from build123d import *

# Parameters (mm, degrees)
SKETCH_1_R      = 7.5
SKETCH_1_R_2    = 5
EXTRUDE_1_DEPTH = 4
SKETCH_2_R      = 8.25
SKETCH_2_R_2    = 7.5
EXTRUDE_2_DEPTH = 0.8
CHAMFER_1_SIZE  = 0.2


with BuildPart() as part:
    # 草图1 → 凸台-拉伸1 (new body)
    with BuildSketch(Plane.XY):
        Circle(SKETCH_1_R)
        Circle(SKETCH_1_R_2, mode=Mode.SUBTRACT)
    extrude(amount=EXTRUDE_1_DEPTH)

    # 草图2 → 凸台-拉伸2 (add)
    with BuildSketch(Plane(origin=(0, 0, 0), x_dir=(-1, 0, 0), z_dir=(0, 0, -1))):
        Circle(SKETCH_2_R)
        Circle(SKETCH_2_R_2, mode=Mode.SUBTRACT)
    extrude(amount=-EXTRUDE_2_DEPTH)

    # 倒角1
    chamfer_1_edges = [part.edges().sort_by_distance(p)[0] for p in [
        (8.25, 0, 0.8),
        (8.25, 0, 0),
        (-7.5, 0, 4),
        (-5, 0, 0),
        (-5, 0, 4),
    ]]
    chamfer(chamfer_1_edges, length=CHAMFER_1_SIZE)


solid = part.part
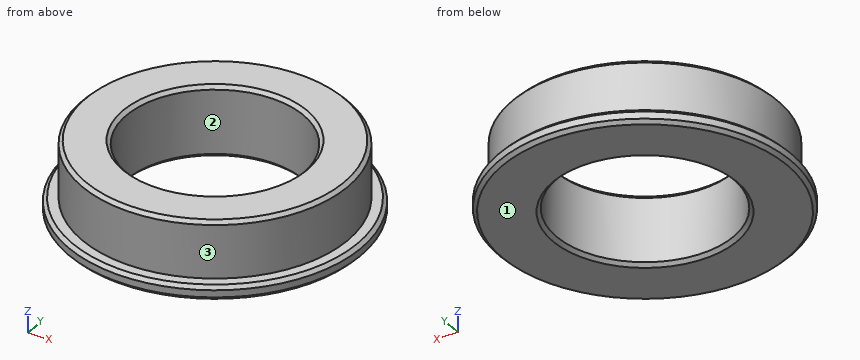
CAD build for the part. Positions are in the model's coordinates, mm. Face numbers are marked on the shaded views. Round coordinates to 2 decimals unless told otherwise and drop trailing zeros. Order: outer loops, then holes, each group sorted by start corner. A loop starts at its lowest first (then second) coordinate and runs counter-clockwise, first axis right, second up. Notation, with made-up numbers: (56.5, -4.5) -> (72.5, -4.5) arc R22 ccw to (72.5, 33.5) -> close; hole circle Ø7 at (21.5, 7). An arc over 180 degrees is marked (long way). Write item = value, one per line. Start each with the question number.
(1) Cut at A-A, the plane x = 0. List the corners of the cut face in (y, z).
(2) Pin check, flat tips, straight feed: P1, Ø1.5, axis at x = 0.5, z = 2.5, coming from the +Y side; P2, Ø8, axis at x = 0, y = 0, coming from the +Z side; P3, Ø2, axis at x = 1.5, z = 1, coming from the +Y side. Stop position of each tip, or through.
(3) Pull direction X, two halves, no side cores. Call the marked faces 1, 2 and 3: released by +X, released by -X, zero draft, split by the parting line, or undercut.
(4) Cut at C-C, the plane z = 1.1. List the corners of the cut face in (x, y).
(5) Probe line 1 (Y direction, x = 0, z = 1.2); line 2 (X direction, y = -3.25, z = 2.95); line 3 (X direction, y = -1, z = 2). List the from-to ranges inside material, lowest first. Write a range as [from, to].
Model answer:
q1.outline = (-8.25, 0.2) -> (-8.05, 0) -> (-5.2, 0) -> (-5, 0.2) -> (-5, 3.8) -> (-5.2, 4) -> (-7.3, 4) -> (-7.5, 3.8) -> (-7.5, 0.8) -> (-8.05, 0.8) -> (-8.25, 0.6) -> close; (5, 0.2) -> (5.2, 0) -> (8.05, 0) -> (8.25, 0.2) -> (8.25, 0.6) -> (8.05, 0.8) -> (7.5, 0.8) -> (7.5, 3.8) -> (7.3, 4) -> (5.2, 4) -> (5, 3.8) -> close
q2.P1 = 7.5
q2.P2 = through
q2.P3 = 8.23
q3.face_1 = zero draft
q3.face_2 = undercut
q3.face_3 = split by the parting line
q4.outline = circle Ø15 at (0, 0); hole circle Ø10 at (0, 0)
q5.line_1 = [-7.5, -5], [5, 7.5]
q5.line_2 = [-6.76, -3.8], [3.8, 6.76]
q5.line_3 = [-7.43, -4.9], [4.9, 7.43]
